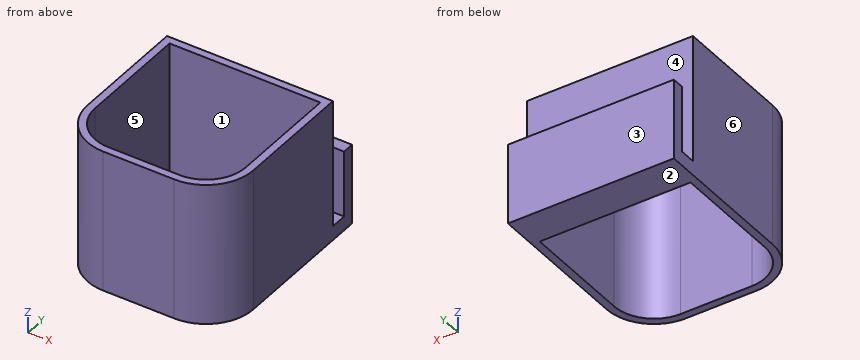
```python
from build123d import *

# Parameters (mm, degrees)
F1_DEPTH = 30
F2_T     = -1.6
F0_W     = 35
F0_H     = 3.5
F3_DEPTH = 3
F0_H_2   = 2.5
F4_DEPTH = 17
F5_DEPTH = 5


with BuildPart() as f1:
    # F0 (on Top) → F1 (new body)
    with BuildSketch(Plane.XY):
        with BuildLine():
            Line((35, -6), (0, -6))
            Line((0, -6), (0, -31))
            ThreePointArc((0, -31), (2.9289321881, -38.0710678119), (10, -41))
            Line((10, -41), (25, -41))
            ThreePointArc((25, -41), (32.0710678119, -38.0710678119), (35, -31))
            Line((35, -31), (35, -6))
        make_face()
    extrude(amount=F1_DEPTH)

    # F2
    f2_openings = [f1.faces().sort_by_distance(p)[0] for p in [
        (17.5, -22.945692, 30),
    ]]
    offset(amount=F2_T, openings=f2_openings)

    # F0 (on Top) → F3 (join)
    with BuildSketch(Plane.XY):
        with Locations((17.5, -4.25)):
            Rectangle(F0_W, F0_H)
    extrude(amount=F3_DEPTH)

    # F0 (on Top) → F4 (join)
    with BuildSketch(Plane.XY):
        with Locations((17.5, -1.25)):
            Rectangle(F0_W, F0_H_2)
    extrude(amount=F4_DEPTH)

    # F5 (cut): a face of the model
    f5_faces = [f1.faces().sort_by_distance(p)[0] for p in [
        (17.5, -23.0670520916, 1.6),
    ]]
    extrude(f5_faces, amount=-F5_DEPTH, mode=Mode.SUBTRACT)


solid = f1.part
```
Source: CAD feature listing. Evaluate the final solid. Frame: model axes, mm. Face numbers are marked on the shaded views. A direction names the side the tool comes from. Round coordinates to 2 decimals unless told otherwise and drop trailing zeros. Loops run counter-clockwise (first coordinate to the right, second up) from the corner with the lowest first, then second, coordinate; pieces in that order, holes last. Notation, with made-up numbers: (86.5, 70.25) - (136.5, 70.25) arc R15 ccw to (136.5, 75.25) - close; hole circle Ø2 at (37.5, -13). An arc over 180 degrees is marked (long way). Use CSV: the item, a comma, the result in double quotes.
Q1. Section query D-D, the plane z = 20. Output: boundary loops of the cut face in (x, y).
Reported:
outline,"(0, -31) arc R10 ccw to (10, -41) - (25, -41) arc R10 ccw to (35, -31) - (35, -6) - (0, -6) - close; hole (1.6, -31) arc R8.4 ccw to (10, -39.4) - (25, -39.4) arc R8.4 ccw to (33.4, -31) - (33.4, -7.6) - (1.6, -7.6) - close"
Q2. Mould query, pull axis Y, two halves, no side actions, for the marked faces 1, 2 and 3. Classes: pulls with the +Y half, pulls with the -Y half, needs draft (parallel to the pull), parting line crosses it, or undercut.
Reported:
face 1,"undercut"
face 2,"needs draft"
face 3,"pulls with the +Y half"
Q3. Section query A-A, the plane z = 11. Output: boundary loops of the cut face in (x, y), then the cut area to 3 significant figures.
Reported:
outline,"(0, -31) arc R10 ccw to (10, -41) - (25, -41) arc R10 ccw to (35, -31) - (35, -6) - (0, -6) - close; (0, -2.5) - (35, -2.5) - (35, 0) - (0, 0) - close; hole (1.6, -31) arc R8.4 ccw to (10, -39.4) - (25, -39.4) arc R8.4 ccw to (33.4, -31) - (33.4, -7.6) - (1.6, -7.6) - close"
area,"289 mm^2"
Q4. Reachability of the marked faces 4, 5 and 6 from +Z, -Z, +X, -X, +Y, -Y: full face, straight path, thin tool, end or side. Return the list, or none.
Reported:
face 4,"+Z, +X, -X"
face 5,"+Z, -Z"
face 6,"+Z, -Z, -X, +Y, -Y"
Q5. Pin query (flat end, axial travel): pin 1 Ø8 at (y, z) = (-33.5, 13) entering from +X; pin 2 Ø1.8 at (x, y) = (25, -4.5) entering from +Z; pin 3 Ø3 at (x, y) = (13, -1) entering from +Z. Return the tip coordinate at first contact, or that it passes through.
Reported:
pin 1,"x = 35"
pin 2,"z = 3"
pin 3,"z = 17"
Q6. Section query C-C, the plane x = 22. Output: boundary loops of the cut face in (y, z).
Reported:
outline,"(-41, 0) - (-39.4, 0) - (-39.4, 30) - (-41, 30) - close; (-7.6, 0) - (0, 0) - (0, 17) - (-2.5, 17) - (-2.5, 3) - (-6, 3) - (-6, 30) - (-7.6, 30) - close"
Q7. Ray query, line 1 along Y through (x, z) = (10, 7.75); line 2 along X through (y, z) = (-13.5, 13.5); line 3 along Y through (x, z) = (29, 8.75). Return the intervals inside material, ascending.
Reported:
line 1,"-41 to -39.4, -7.6 to -6, -2.5 to 0"
line 2,"0 to 1.6, 33.4 to 35"
line 3,"-40.17 to -38.39, -7.6 to -6, -2.5 to 0"
Q8. Section query B-B, the plane y = -23. Output: boundary loops of the cut face in (x, z).
Reported:
outline,"(0, 0) - (1.6, 0) - (1.6, 30) - (0, 30) - close; (33.4, 0) - (35, 0) - (35, 30) - (33.4, 30) - close"
